For this review, take the finished solid that the model builds, in its own axes (mm). Face numbers are marked on the shaded views. A direction names the side the tool comes from. Coordinates: 2 decimals unless noted, no trailing zeros. Order: outer loops, then holes, each group sorted by start corner. A loop starts at its lowest first (then second) coordinate and runs counter-clockwise, first axis right, second up.
from build123d import *

# Parameters (mm, degrees)
F1_DEPTH = 57.15
F3_DEPTH = 44.45
F4_R     = 12.7
F5_DEPTH = 44.45
F6_R     = 5.08
F7_DEPTH = 25.4


with BuildPart() as f1:
    # F0 (on Front) → F1 (new body)
    with BuildSketch(Plane.XZ):
        Polygon((-31.75, 0), (0, 0), (31.75, 0), (31.75, 12.70301), (12.7, 12.70301), (12.7, 21.59), (63.5, 21.59), (63.5, 85.09), (0, 85.09), (-63.5, 85.09), (-63.5, 21.59), (-12.7, 21.59), (-12.7, 12.70301), (-31.75, 12.70301), align=None)
    extrude(amount=F1_DEPTH)

    # F2 (on face) → F3 (cut)
    with BuildSketch(Plane.XZ.offset(57.15)):
        with BuildLine():
            Line((-63.5, 85.09), (-63.5, 34.29))
            Line((-63.5, 34.29), (-47.625, 34.29))
            Line((-47.625, 34.29), (-21.093426, 73.840173))
            ThreePointArc((-21.093426, 73.840173), (-11.952941, 82.101765), (0, 85.09))
            Line((0, 85.09), (-63.5, 85.09))
        make_face()
        with BuildLine():
            Line((63.5, 85.09), (0, 85.09))
            ThreePointArc((0, 85.09), (11.952941, 82.101765), (21.093426, 73.840173))
            Line((21.093426, 73.840173), (47.625, 34.29))
            Line((47.625, 34.29), (63.5, 34.29))
            Line((63.5, 34.29), (63.5, 85.09))
        make_face()
    extrude(amount=-F3_DEPTH, mode=Mode.SUBTRACT)

    # F4 (on face) → F5 (cut)
    with BuildSketch(Plane.XZ.offset(57.15)):
        with Locations((0, 66.04)):
            Circle(F4_R)
    extrude(amount=-F5_DEPTH, mode=Mode.SUBTRACT)

    # F6 (on face) → F7 (cut)
    with BuildSketch(Plane.XY.offset(85.09)):
        with Locations((0, -34.925)):
            Circle(F6_R)
    extrude(amount=-F7_DEPTH, mode=Mode.SUBTRACT)


solid = f1.part
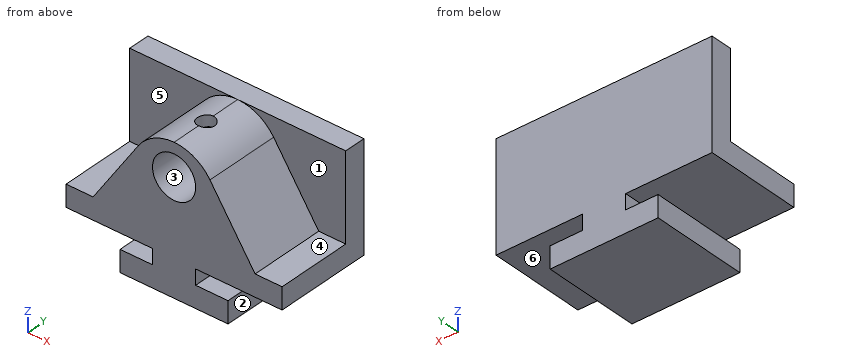
1. Machinability: for the marked faces 1, 2 and 3, which of the approach directions +Z, -Z, +X, -X, +Y, -Y give a long, thin tool a straight path to every point of the face, cutting with its end or side? Answer none if there is none.
Answer below:
face 1: +Z, +X, -Y
face 2: -Z, +X, +Y, -Y
face 3: -Y
2. Take a section at A-A, the plane y = -6. Give the boundary of the cut face in (x, z).
Answer below:
outline: (-63.5, 21.59) - (-12.7, 21.59) - (-12.7, 12.7) - (-31.75, 12.7) - (-31.75, 0) - (31.75, 0) - (31.75, 12.7) - (12.7, 12.7) - (12.7, 21.59) - (63.5, 21.59) - (63.5, 85.09) - (-63.5, 85.09) - close
3. Clearance check with flat-ended pins moving along their axes: pin 1 Ø8 at (x, y) = (15.5, -40.5) entering from +Z; pin 2 Ø14 at (y, z) = (-41, 9) entering from -X; pin 3 Ø23 at (x, z) = (0, 66.04) entering from -Y. State where each tip first meets the part, or that it passes through.
Answer below:
pin 1: stops at z = 82.34
pin 2: stops at x = -31.75
pin 3: stops at y = -12.7
4. Take a section at D-D, the plane x = -38.5. Give the boundary of the cut face in (y, z), plus the area to 3 significant figures.
Answer below:
outline: (-57.15, 21.59) - (0, 21.59) - (0, 85.09) - (-12.7, 85.09) - (-12.7, 47.89) - (-57.15, 47.89) - close
area: 1,980 mm2
5. Take a section at C-C, the plane z = 45. Give the boundary of the cut face in (x, y), plus the area to 3 significant figures.
Answer below:
outline: (-63.5, -12.7) - (-40.44, -12.7) - (-40.44, -57.15) - (40.44, -57.15) - (40.44, -12.7) - (63.5, -12.7) - (63.5, 0) - (-63.5, 0) - close
area: 5,210 mm2
6. The part is to be moulded in two halves that separate along Z. For the marked faces 4, 5 and 6, say which applies: +Z half, -Z half, draft (parallel to the pull), parting line (faces both ways), or undercut.
Answer below:
face 4: +Z half
face 5: draft
face 6: undercut
7. To check wall thickness, follow L1, parallel to Y at x = 0, z = 82.5 (3 decimals); L2, parallel to Z at x = 31, y = -7; L3, parallel to Y at x = 43.5, z = 80.5. State the ranges of each line that lie inside material, in increasing order.
Answer below:
L1: y = -57.15 to -40.005, -29.845 to 0
L2: z = 0 to 12.7, 21.59 to 85.09
L3: y = -12.7 to 0
8. Take a section at B-B, the plane x = -19.5. Give the boundary of the cut face in (y, z), plus the area to 3 significant figures.
Answer below:
outline: (-57.15, 0) - (0, 0) - (0, 12.7) - (-57.15, 12.7) - close; (-57.15, 21.59) - (0, 21.59) - (0, 85.09) - (-12.7, 85.09) - (-12.7, 75.97) - (-57.15, 75.97) - close
area: 3,950 mm2
